```python
from build123d import *

# Parameters (mm, degrees)
SKETCH_1_W          = 42
SKETCH_1_H          = 42
EXTRUDE_1_DEPTH     = 2
SKETCH_2_R          = 1.5
SKETCH_2_R_2        = 1.25
SKETCH_2_W          = 8.5
SKETCH_2_H          = 16
SKETCH_2_W_2        = 22
SKETCH_2_H_2        = 9
CUT_EXTRUDE_1_DEPTH = 2
FILLET_1_R          = 3
SKETCH_3_R          = 3
SKETCH_3_R_2        = 1.25
SKETCH_3_R_3        = 1.234283691
SKETCH_3_R_4        = 1.239522306
EXTRUDE_2_DEPTH     = 6


with BuildPart() as part:
    # 草图1 → 凸台-拉伸1 (new body)
    with BuildSketch(Plane.XY):
        Rectangle(SKETCH_1_W, SKETCH_1_H)
    extrude(amount=EXTRUDE_1_DEPTH)

    # 草图2 → 切除-拉伸1 (cut)
    with BuildSketch(Plane(origin=(0, 0, 0), x_dir=(-1, 0, 0), z_dir=(0, 0, -1))):
        with Locations((-6.25, 15)):
            Circle(SKETCH_2_R)
        with Locations((6.25, 15)):
            Circle(SKETCH_2_R)
        with Locations((6.25, -5)):
            Circle(SKETCH_2_R)
        with Locations((-6.25, -5)):
            Circle(SKETCH_2_R)
        with Locations((18, -18)):
            Circle(SKETCH_2_R_2)
        with Locations((-18, -18)):
            Circle(SKETCH_2_R_2)
        with Locations((-18, 18)):
            Circle(SKETCH_2_R_2)
        with Locations((18, 18)):
            Circle(SKETCH_2_R_2)
        with Locations((0, 5)):
            Rectangle(SKETCH_2_W, SKETCH_2_H)
        with Locations((0, -12.5)):
            Rectangle(SKETCH_2_W_2, SKETCH_2_H_2)
    extrude(amount=-CUT_EXTRUDE_1_DEPTH, mode=Mode.SUBTRACT)

    # 圆角1
    fillet_1_edges = [part.edges().sort_by_distance(p)[0] for p in [
        (-11, -8, 1),
        (-11, -17, 1),
        (11, -17, 1),
        (11, -8, 1),
        (4.25, 13, 1),
        (-4.25, 13, 1),
        (-4.25, -3, 1),
        (4.25, -3, 1),
        (21, -21, 1),
        (-21, -21, 1),
        (-21, 21, 1),
        (21, 21, 1),
    ]]
    fillet(fillet_1_edges, radius=FILLET_1_R)

    # 草图3 → 凸台-拉伸2 (add)
    # profile 1 of 4: a face of its own
    with BuildSketch(Plane(origin=(0, 0, 0), x_dir=(-1, 0, 0), z_dir=(0, 0, -1))):
        with Locations((18, 18)):
            Circle(SKETCH_3_R)
        with Locations((18, 18)):
            Circle(SKETCH_3_R_2, mode=Mode.SUBTRACT)
    # profile 2 of 4: a face of its own
    with BuildSketch(Plane(origin=(0, 0, 0), x_dir=(-1, 0, 0), z_dir=(0, 0, -1))):
        with Locations((18, -18)):
            Circle(SKETCH_3_R)
        with Locations((18, -18)):
            Circle(SKETCH_3_R_2, mode=Mode.SUBTRACT)
    # profile 3 of 4: a face of its own
    with BuildSketch(Plane(origin=(0, 0, 0), x_dir=(-1, 0, 0), z_dir=(0, 0, -1))):
        with Locations((-18, -18)):
            Circle(SKETCH_3_R)
        with Locations((-18, -18)):
            Circle(SKETCH_3_R_3, mode=Mode.SUBTRACT)
    # profile 4 of 4: a face of its own
    with BuildSketch(Plane(origin=(0, 0, 0), x_dir=(-1, 0, 0), z_dir=(0, 0, -1))):
        with Locations((-18, 18)):
            Circle(SKETCH_3_R)
        with Locations((-18, 18)):
            Circle(SKETCH_3_R_4, mode=Mode.SUBTRACT)
    extrude(amount=EXTRUDE_2_DEPTH)


solid = part.part
```
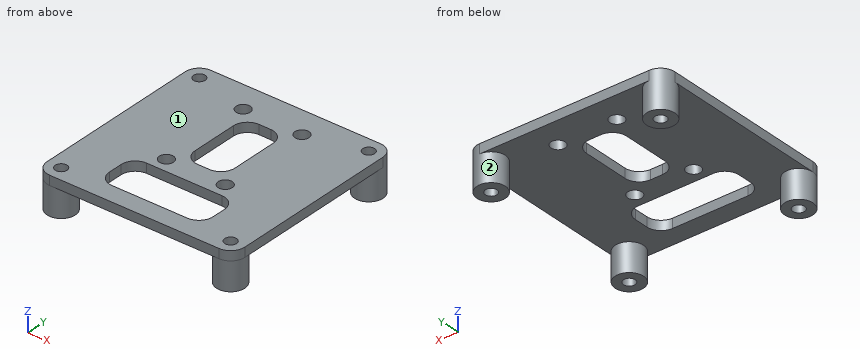
Geometry check sheet. Reference: the model listing, model coordinates, mm. Face numbers are marked on the shaded views. Coordinates: 2 decimals unless noted, no trailing zeros. Order: outer loops, then holes, each group sorted by start corner. A loop starts at its lowest first (then second) coordinate and runs counter-clockwise, first axis right, second up. Notation, with made-up numbers: (44.25, 43) - (91.25, 43) arc R13 ccw to (91.25, 52) - close; hole circle Ø1 at (-7, 17.25). An arc over 180 degrees is marked (long way). Use one line per item in the form item = value.
1. Section check A-A (z = -0.75). Record the boundary of the cut face in (x, y).
Here are the results:
outline = circle Ø6 at (-18, -18); circle Ø6 at (-18, 18); circle Ø6 at (18, -18); circle Ø6 at (18, 18); hole circle Ø2.5 at (-18, -18); hole circle Ø2.5 at (-18, 18); hole circle Ø2.48 at (18, 18); hole circle Ø2.47 at (18, -18)
2. Section check D-D (x = 10.5). Record the boundary of the cut face in (y, z).
Here are the results:
outline = (-21, 0) - (-15.66, 0) - (-15.66, 2) - (-21, 2) - close; (-9.34, 0) - (21, 0) - (21, 2) - (-9.34, 2) - close
3. Gauge pin test, flat end, axial feed: pin 1 (3.5 mm diameter, centred on x = 6.25, y = 15, fed in from -Z). Record the tip position at first contact, or that the pin passes through.
Here are the results:
pin_1 = 0
4. Section check C-C (y = 5). Record the boundary of the cut face in (x, z), then the cut area to 3 significant figures.
Here are the results:
outline = (-21, 0) - (-4.25, 0) - (-4.25, 2) - (-21, 2) - close; (4.25, 0) - (21, 0) - (21, 2) - (4.25, 2) - close
area = 67.0 mm²
5. Scan lines: line 1 (Y direction, x = -6.25, z = 1.25); line 2 (Y direction, x = -18, z = -2.75); line 3 (Z direction, x = 14, y = -8). Record each from-to range of solid material in increasing order.
Here are the results:
line_1 = -21 to -17, -8 to -6.5, -3.5 to 13.5, 16.5 to 21
line_2 = -21 to -19.25, -16.75 to -15, 15 to 16.75, 19.25 to 21
line_3 = 0 to 2
6. Section check B-B (x = -6.25). Record the boundary of the cut face in (y, z), then the cut area to 3 significant figures.
Here are the results:
outline = (-21, 0) - (-17, 0) - (-17, 2) - (-21, 2) - close; (-8, 0) - (-6.5, 0) - (-6.5, 2) - (-8, 2) - close; (-3.5, 0) - (13.5, 0) - (13.5, 2) - (-3.5, 2) - close; (16.5, 0) - (21, 0) - (21, 2) - (16.5, 2) - close
area = 54.0 mm²
7. Draft check along Y on the marked faces 1 and 2. Enter one of: pulls with the +Y half, pulls with the -Y half, needs draft (parallel to the pull), parting line crosses it, or undercut.
Here are the results:
face_1 = needs draft
face_2 = undercut
